Input: dimensioned drawing with shaded views. Units: mm. Origin: part minimum x, y, z. A direction names the side the tool comes from. Give positions to 0.01 mm unless a question says otherwise; leave off trailing zeros. Loops run counter-clockwise (first coordinate to the right, second up) from the corner with the lowest first, then second, coordinate; pieces in that order, holes last. Notation, with made-up numbers: M 18.25,-29.5 L 69.25,-29.5 A22 ccw 69.25,-8.5 Z; hole C -18.75,78 d2. An arc over 180 degrees is marked long. Answer in a Markdown table with one row per item.
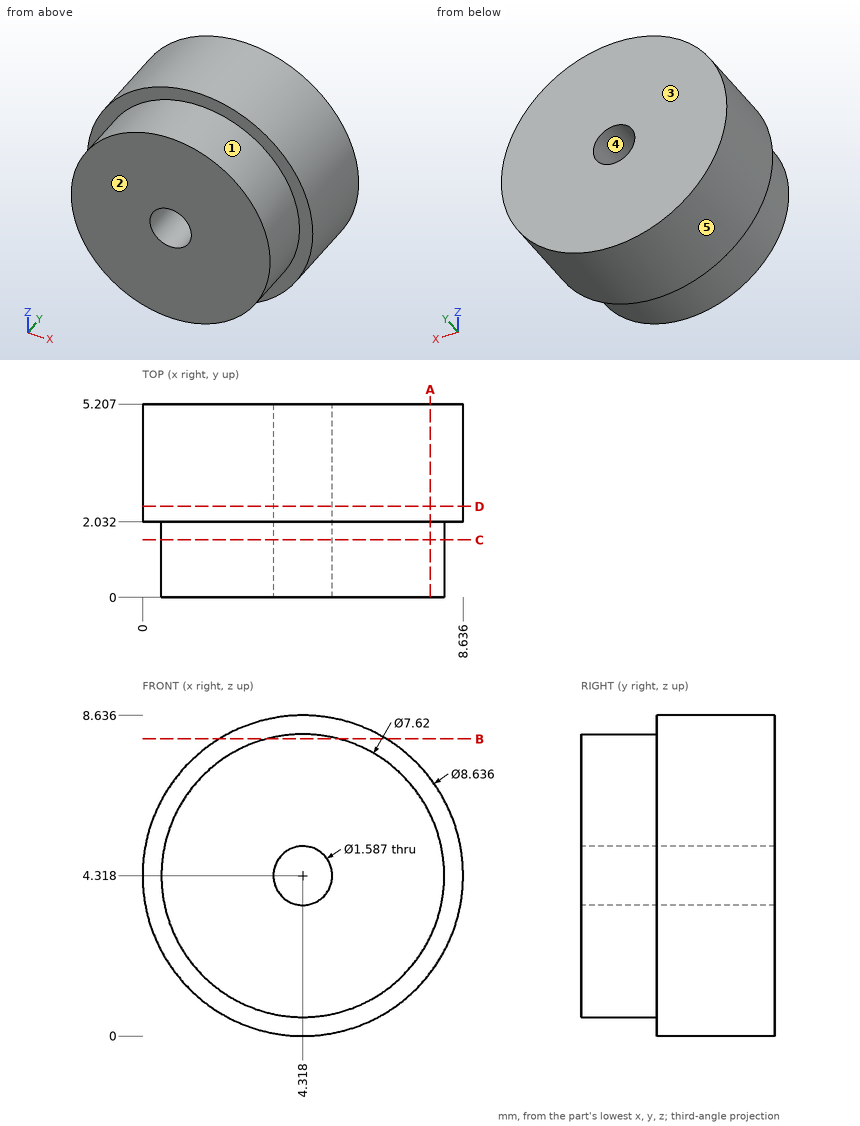
Q1. Reachability of the marked faces 1 and 2 from +Z, -Z, +X, -X, +Y, -Y: full face, straight path, thin tool, end or side. Return the list, or none.
Values follow:
| item | result |
|---|---|
| face 1 | -Y |
| face 2 | +Z, -Z, +X, -X, -Y |
Q2. Section query C-C (y = 1.55). Output: boundary loops of the cut face in (x, z).
Values follow:
| item | result |
|---|---|
| outline | C 4.32,4.32 d7.62; hole C 4.32,4.32 d1.59 |
Q3. Mould query, pull axis Z, two halves, no side actions, for the marked faces 3, 4 and 5. Classes: +Z half, -Z half, draft (parallel to the pull), parting line (faces both ways), or undercut.
Values follow:
| item | result |
|---|---|
| face 3 | draft |
| face 4 | undercut |
| face 5 | parting line |
Q4. Section query A-A (x = 7.75). Output: boundary loops of the cut face in (y, z).
Values follow:
| item | result |
|---|---|
| outline | M 0,2.66 L 2.03,2.66 L 2.03,1.7 L 5.21,1.7 L 5.21,6.94 L 2.03,6.94 L 2.03,5.97 L 0,5.97 Z |
Q5. Contact query for a flat-ended pin moving along its axis: pin 1 Ø1.5 at (y, z) = (3, 7.5) entering from -X. Output: stop coordinate, or through.
Values follow:
| item | result |
|---|---|
| pin 1 | x = 0.75 |
Q6. Section query B-B (z = 8). Output: boundary loops of the cut face in (x, y).
Values follow:
| item | result |
|---|---|
| outline | M 2.06,2.03 L 3.34,2.03 L 3.34,0 L 5.3,0 L 5.3,2.03 L 6.57,2.03 L 6.57,5.21 L 2.06,5.21 Z |
Q7. Ray query, probe 1 along X at (y, z) = (1.75, 4.25); probe 2 along Z at (x, y) = (4, 0.75) (1 decimal); probe 3 along Z at (x, y) = (3.75, 4.7) (1 decimal). Return the intervals inside material, ascending. Write a range as from..to.
Values follow:
| item | result |
|---|---|
| probe 1 | 0.51..3.53, 5.11..8.13 |
| probe 2 | 0.5..3.6, 5..8.1 |
| probe 3 | 0..3.8, 4.9..8.6 |
Q8. Section query D-D (y = 2.45). Output: boundary loops of the cut face in (x, z) (1 decimal), plus the area to 3 significant figures.
Values follow:
| item | result |
|---|---|
| outline | C 4.3,4.3 d8.6; hole C 4.3,4.3 d1.6 |
| area | 56.6 mm^2 |
